```python
from build123d import *

# Parameters (mm, degrees)
BOSS_EXTRUDE1_DEPTH = 50
SKETCH3_R           = 9
CUT_EXTRUDE1_DEPTH  = 50
SKETCH4_R           = 13.05
CUT_EXTRUDE2_DEPTH  = 5
SKETCH6_R           = 2.2
CUT_EXTRUDE3_DEPTH  = 8


with BuildPart() as part:
    # Sketch1 → Boss-Extrude1 (new body)
    with BuildSketch(Plane(origin=(0, 0, 0), x_dir=(0, 0, -1), z_dir=(1, 0, 0))):
        Polygon((0, 0), (38, 0), (38, 38), (31.6, 38), (31.6, 6.4), (0, 6.4), align=None)
    extrude(amount=BOSS_EXTRUDE1_DEPTH)

    # Sketch3 → Cut-Extrude1 (cut)
    with BuildSketch(Plane(origin=(0, 0, -38), x_dir=(-1, 0, 0), z_dir=(0, 0, -1))):
        with Locations((-25, 17.5)):
            Circle(SKETCH3_R)
    extrude(amount=-CUT_EXTRUDE1_DEPTH, mode=Mode.SUBTRACT)

    # Sketch4 → Cut-Extrude2 (cut)
    with BuildSketch(Plane(origin=(0, 0, -38), x_dir=(-1, 0, 0), z_dir=(0, 0, -1))):
        with Locations((-25, 17.5)):
            Circle(SKETCH4_R)
    extrude(amount=-CUT_EXTRUDE2_DEPTH, mode=Mode.SUBTRACT)

    # Sketch6 → Cut-Extrude3 (cut)
    with BuildSketch(Plane(origin=(0, 6.4, 0), x_dir=(1, 0, 0), z_dir=(0, 1, 0))):
        with Locations(Location((9.217627347, 16, 0), (0, 0, 270))):
            Circle(SKETCH6_R)
        with Locations(Location((45.217627347, 16, 0), (0, 0, 270))):
            Circle(SKETCH6_R)
    extrude(amount=-CUT_EXTRUDE3_DEPTH, mode=Mode.SUBTRACT)


solid = part.part
```
CAD build for the part. Positions are in the model's coordinates, mm. A direction names the side the tool comes from. Coordinates: 2 decimals unless noted, no trailing zeros. Order: outer loops, then holes, each group sorted by start corner. A loop starts at its lowest first (then second) coordinate and runs counter-clockwise, first axis right, second up. Notation, with made-up numbers: (-36, 80) - (-1, 80) arc R16 cw to (-1, 100) - close; hole circle Ø8 at (72, 15.5). An arc over 180 degrees is marked (long way). Use a Markdown table: item, result. Add a question column.
(1) Saw through at C-C (y = 23). Give the cut face in (x, z).
(2) Saw through at B-B (z = -16). Give the cut face in (x, y).
(3) Drill centre lines: line 1 along X through (y, z) = (5.25, -16); line 2 along X through (y, z) = (17, -32); line 3 along Y through (x, z) = (14, -23). Where is each one in solid material? Low to high. Write a range as [from, to].
(4) Saw through at A-A (x = 25). Give the cut face in (y, z), then the cut area to 3 significant figures.
(5) Saw through at D-D (x = 4). Give the cut face in (y, z).
(6) Flat gauge pins, fed straight in: pin 1 (4 mm diameter, centred on x = 5.5, z = -7, fed in from +Y); pin 2 (2 mm diameter, centred on x = 14, y = 8, fed in from +Z); pin 3 (14.5 mm diameter, centred on x = 25, y = 17.5, fed in from +Z); pin 4 (1.5 mm diameter, centred on x = 19, z = -9.5, fed in from -Y). Where does each tip first touch, or does it go through?
(7) Pull direction Z, two halves, no side cores. Call faces 1 (the face through (43.07, 3.24, -16.48)), 2 (the face through (16, 21, -33)), 3 (the face through (8.375, 3.245, -13.968)), 4 (the face through (16.416, 20.203, -32.31)): +Z half, -Z half, draft (parallel to the pull), parting line (faces both ways), or undercut.
(8) Which spindle directions (+Z, -Z, +X, -X, +Y, -Y) get a long thin tool onto all of the face, cutting with end or side? Do faces 5 (the face through (25, 3, 0)), 6 (the face through (18.98, 5.92, -35.53)), 7 (the face through (25, 6.4, -16)). Say none if no direction does.
Solved:
| question | item | result |
|---|---|---|
| 1 | outline | (0, -38) - (13.17, -38) - (13.17, -33) - (17.88, -33) - (17.88, -31.6) - (0, -31.6) - close; (32.12, -33) - (36.83, -33) - (36.83, -38) - (50, -38) - (50, -31.6) - (32.12, -31.6) - close |
| 2 | outline | (0, 0) - (7.02, 0) - (7.02, 6.4) - (0, 6.4) - close; (11.42, 0) - (43.02, 0) - (43.02, 6.4) - (11.42, 6.4) - close; (47.42, 0) - (50, 0) - (50, 6.4) - (47.42, 6.4) - close |
| 3 | line 1 | x = [0, 7.02], [11.42, 43.02], [47.42, 50] |
| 3 | line 2 | x = [0, 16.01], [33.99, 50] |
| 3 | line 3 | y = [0, 6.4] |
| 4 | outline | (0, -38) - (4.45, -38) - (4.45, -33) - (8.5, -33) - (8.5, -31.6) - (6.4, -31.6) - (6.4, 0) - (0, 0) - close; (26.5, -33) - (30.55, -33) - (30.55, -38) - (38, -38) - (38, -31.6) - (26.5, -31.6) - close |
| 4 | area | 290 mm² |
| 5 | outline | (0, -38) - (38, -38) - (38, -31.6) - (6.4, -31.6) - (6.4, 0) - (0, 0) - close |
| 6 | pin 1 | stops at y = 6.4 |
| 6 | pin 2 | stops at z = -31.6 |
| 6 | pin 3 | passes through |
| 6 | pin 4 | stops at y = 0 |
| 7 | face 1 | undercut |
| 7 | face 2 | -Z half |
| 7 | face 3 | undercut |
| 7 | face 4 | draft |
| 8 | face 5 | +Z, +X, -X, +Y, -Y |
| 8 | face 6 | -Z |
| 8 | face 7 | +Z, +X, -X, +Y |
